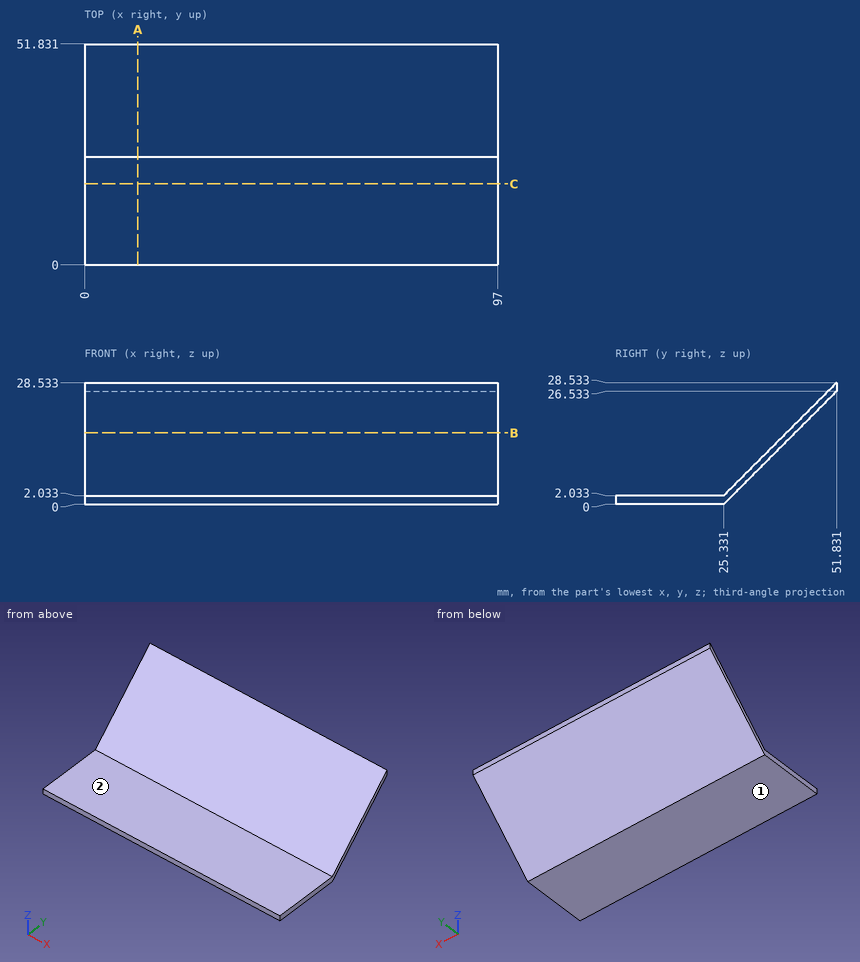
Can you work these out from the drawing? Everything is in mm from the part's minimum corner. A direction names the side the tool comes from. Coordinates: 2 decimals unless noted, no trailing zeros. Loops run counter-clockwise (first coordinate to the right, second up) from the corner with the lowest first, then second, coordinate; pieces in that order, holes last.
1. Imagine slicing it at A-A, the plane x = 12.5. Please give me the cut outline in (y, z).
2. I need wall thicknesses on L1, parallel to Z at x = 36, y = 23; L2, parallel to Y at x = 7.5, z = 16; L3, parallel to Z at x = 87.5, y = 31. Which ranges of each line are inside material? Lowest first, please.
3. Imagine slicing it at B-B, the plane z = 16.75. Please give me the cut outline in (x, y), and give its area (3 significant figures).
4. For the marked faces 1 and 2, which set-ups out of +Z, -Z, +X, -X, +Y, -Y let a thin tool reach every point of the face, with its end or its side?
5. For P1, Ø2, axis at x = 64, z = 21.5, coming from the +Y side; P2, Ø5, axis at x = 33, z = 16, coming from the +Y side; P3, Ø4, axis at x = 85.5, z = 7, coming from the -Y side, each with a flat end and sliding along its axis, tell me the tip position at first contact or that it passes through.
6. Imagine slicing it at C-C, the plane y = 19. Please give me the cut outline in (x, z), and give its area (3 significant figures).
Taken from the geometry:
1. outline: (0, 0) - (25.33, 0) - (51.83, 26.53) - (51.83, 28.53) - (25.33, 2.03) - (0, 2.03) - close
2. L1: z = 0 to 2.03
2. L2: y = 39.3 to 41.31
2. L3: z = 5.68 to 7.7
3. outline: (0, 40.05) - (97, 40.05) - (97, 42.06) - (0, 42.06) - close
3. area: 195 mm2
4. face 1: -Z, +X, -X, +Y, -Y
4. face 2: +Z, +X, -X, -Y
5. P1: stops at y = 47.8
5. P2: stops at y = 43.81
5. P3: stops at y = 28.3
6. outline: (0, 0) - (97, 0) - (97, 2.03) - (0, 2.03) - close
6. area: 197 mm2
